Can you work these out from the drawing? Everything is in mm from the part's minimum corner. A direction names the side the tool comes from. Round coordinates to 2 decimals unless told otherwise and drop trailing zeros. Write each loop counter-clockwise with the first axis right and the second up, starting at its lowest first coordinate (ties: lowest second). Pieces come first, ordered by that corner, then holes. Notation, with made-up numbers: (28.25, 47) - (70.25, 47) arc R31 cw to (70.25, 84) - close; hole circle Ø9 at (-36.5, -14.5). An arc over 180 degrees is marked (long way). One line per item, written item: value. Start each with the question number.
(1) I'm going to push flat-ended pins straight in: pin 1 Ø6 at (x, y) = (6.5, 13.5) entering from -Z; pin 2 Ø8 at (y, z) = (19, 20) entering from +X; pin 3 Ø2 at (x, z) = (2, 16.5) entering from +Y; pin 4 Ø1.5 at (x, z) = (10.5, 14.5) entering from -Y. Where does each tip first touch, or does it pass through?
(2) I want a section at B-B on z = 21. List the corners of the cut face in (x, y) for me.
(3) I want a section at C-C on y = 28.1. List the corners of the cut face in (x, z) for me.
(4) If I drill on L1, parallel to Z at x = 5.5, y = 20.5; L2, parallel to Z at x = 12, y = 3.1; L3, parallel to Y at x = 12.75, z = 2 (1 decimal), over which ranges is the centre line in solid material (lowest first)? Write a range as from..to.
(5) On a 3-axis mill with a long thin cutter (end or side, diameter ignored), from which of +Z, -Z, +X, -X, +Y, -Y can I reach the whole of each face in a straight line? I mean the marked faces 1, 2, 3 and 4. Say none if no direction works.
(6) I want a section at A-A on x = 2.25. List the corners of the cut face in (y, z) for me, plus the area to 3 significant figures.
(7) Thinking about a two-plate mould opening in Y: for the marked faces 5, 6 and 7, which applies, +Y half, -Y half, draft (parallel to the pull), parting line (faces both ways), or undercut?
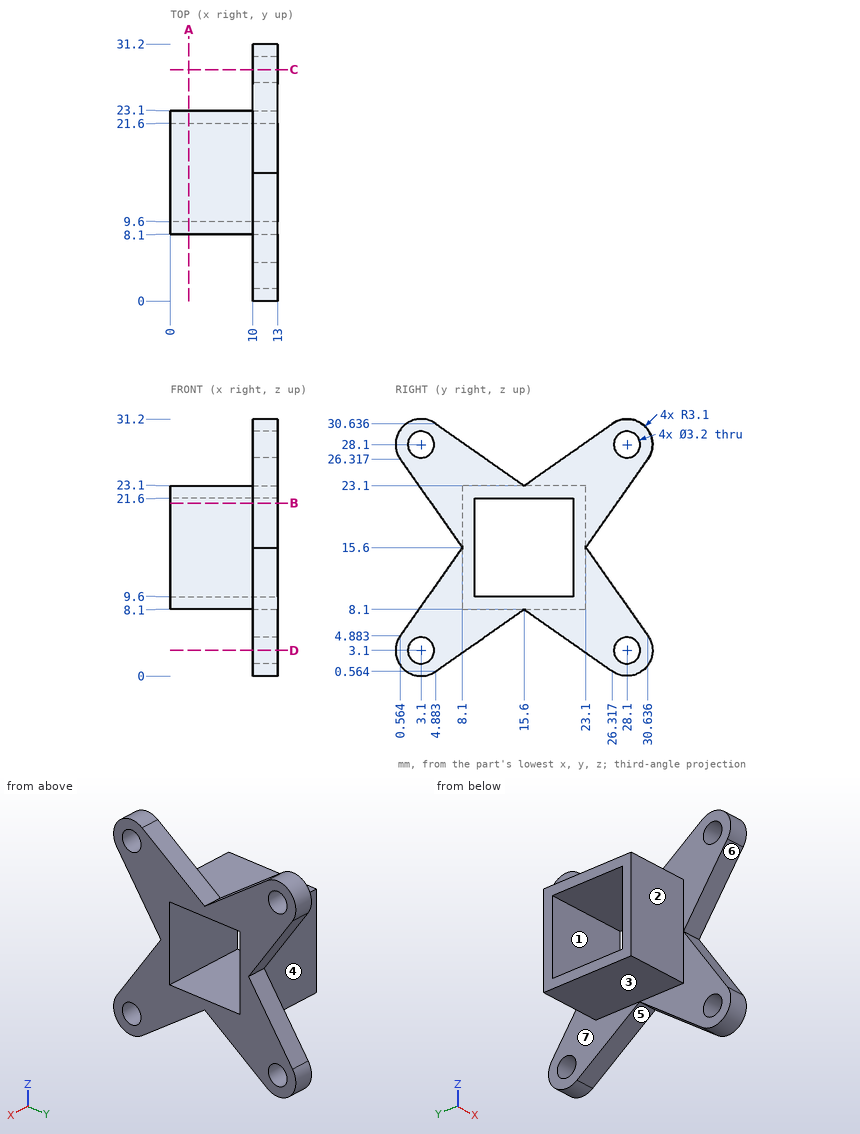
Established:
1. pin 1: z = 8.1
1. pin 2: x = 13
1. pin 3: y = 23.1
1. pin 4: y = 6.8
2. outline: (0, 8.1) - (10, 8.1) - (10, 4.3) - (13, 4.3) - (13, 9.6) - (0, 9.6) - close; (0, 21.6) - (13, 21.6) - (13, 26.9) - (10, 26.9) - (10, 23.1) - (0, 23.1) - close
3. outline: (10, 0) - (13, 0) - (13, 1.5) - (10, 1.5) - close; (10, 4.7) - (13, 4.7) - (13, 8.49) - (10, 8.49) - close; (10, 22.71) - (13, 22.71) - (13, 26.5) - (10, 26.5) - close; (10, 29.7) - (13, 29.7) - (13, 31.2) - (10, 31.2) - close
4. L1: 8.1..9.6, 21.6..23.1
4. L2: 0..1.5, 4.7..8.49, 22.71..26.5, 29.7..31.2
4. L3: 0.2..1.9, 4.3..6.9, 24.3..26.9, 29.3..31
5. face 1: +X, -X
5. face 2: +Z, -Z, -X, -Y
5. face 3: -Z, -X, +Y, -Y
5. face 4: +Z, -Z, -X, +Y
6. outline: (8.1, 8.1) - (23.1, 8.1) - (23.1, 23.1) - (8.1, 23.1) - close; hole (9.6, 9.6) - (21.6, 9.6) - (21.6, 21.6) - (9.6, 21.6) - close
6. area: 81.0 mm2
7. face 5: undercut
7. face 6: -Y half
7. face 7: draft
